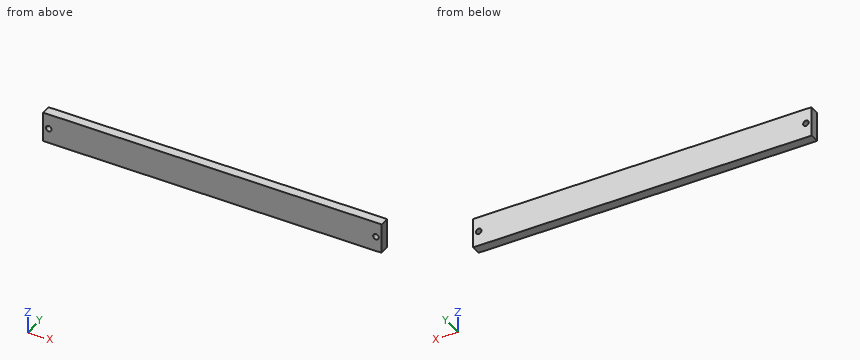
```python
from build123d import *

# Parameters (mm, degrees)
CROQUIS1_W              = 180
CROQUIS1_H              = 16
SALIENTE_EXTRUIR1_DEPTH = 5
CROQUIS2_R              = 1.5
CORTAR_EXTRUIR1_DEPTH   = 91.493093659


with BuildPart() as part:
    # Croquis1 → Saliente-Extruir1 (new body)
    with BuildSketch(Plane(origin=(0, 0, 0), x_dir=(1, 0, 0), z_dir=(0, 1, 0))):
        Rectangle(CROQUIS1_W, CROQUIS1_H)
    extrude(amount=SALIENTE_EXTRUIR1_DEPTH)

    # Croquis2 → Cortar-Extruir1 (cut, through all)
    with BuildSketch(Plane.XZ):
        with Locations(Location((-87, 0, 0), (0, 0, 270))):
            Circle(CROQUIS2_R)
    cortar_extruir1 = extrude(amount=-CORTAR_EXTRUIR1_DEPTH, mode=Mode.SUBTRACT)

    # Simetría1: Cortar-Extruir1 across plane
    add(cortar_extruir1.mirror(Plane(origin=(0, 0, 0), x_dir=(0, 0, 1), z_dir=(1, 0, 0))), mode=Mode.SUBTRACT)


solid = part.part
```
Verification items for the finished model (mm, model axes). Coordinates: 2 decimals unless noted, no trailing zeros. Order: outer loops, then holes, each group sorted by start corner. A loop starts at its lowest first (then second) coordinate and runs counter-clockwise, first axis right, second up. Notation, with made-up numbers: (8, 4) -> (25, 4) arc R34 ccw to (25, 35) -> close; hole circle Ø2 at (64, -3). An arc over 180 degrees is marked (long way). Put each result on its own line as item: value. Start each with the question number.
1) Material ranges on L1, parallel to X at y = 2.4, z = 0; L2, parallel to Z at x = 87, y = 2, recorded low to high.
2) Cross-section at A-A (z = 0). Enter the section's corners in (x, y).
3) Go/stop test with a flat-tipped pin: pin 1 (2.5 mm diameter, centred on x = -87, z = 0, fed in from -Y). Record where the tip stops, or that it passes through.
4) Cross-section at B-B (x = 87). Enter the section's corners in (y, z), plus the area to 3 significant figures.
Geometry check:
1. L1: x = -90 to -88.5, -85.5 to 85.5, 88.5 to 90
1. L2: z = -8 to -1.5, 1.5 to 8
2. outline: (-90, 0) -> (-88.5, 0) -> (-88.5, 5) -> (-90, 5) -> close; (-85.5, 0) -> (85.5, 0) -> (85.5, 5) -> (-85.5, 5) -> close; (88.5, 0) -> (90, 0) -> (90, 5) -> (88.5, 5) -> close
3. pin 1: passes through
4. outline: (0, -8) -> (5, -8) -> (5, -1.5) -> (0, -1.5) -> close; (0, 1.5) -> (5, 1.5) -> (5, 8) -> (0, 8) -> close
4. area: 65.0 mm^2
